Verification items for the finished model (mm, model axes). A direction names the side the tool comes from. Coordinates: 2 decimals unless noted, no trailing zeros. Order: outer loops, then holes, each group sorted by start corner. A loop starts at its lowest first (then second) coordinate and runs counter-clockwise, first axis right, second up. Notation, with made-up numbers: (-3, 35.5) -> (29, 35.5) arc R6 cw to (29, 45.5) -> close; hole circle Ø10 at (42, 59.5). An arc over 180 degrees is marked (long way). Write each question's results on one line, items separated by ' | '. Start each with the question number.
(1) Go/stop test with flat-tipped pins: pin 1 (2 mm diameter, centred on y = -5, z = -49, fed in from -X); pin 2 (2.5 mm diameter, centred on y = -3, z = -60.5, fed in from -X); pin 3 (2.5 mm diameter, centred on y = -5, z = -53, fed in from +X). Record where each tip stops, or that it passes through.
(2) Cross-section at D-D on z = -83.5. Enter the section's corners in (x, y), and give its area (3 significant figures).
(3) Cross-section at B-B on z = -15.5. Enter the section's corners in (x, y), and give its area (3 significant figures).
(4) Cross-section at C-C on x = -59.5. Enter the section's corners in (y, z).
(5) Cross-section at A-A on y = -4.25. Enter the section's corners in (x, z), and give its area (3 significant figures).
(6) Draft check along X on faces 3 (the flat face through (-15.492, -4, -57)), 4 (the cylindrical face through (-2.234, -3.757, -101.575)), 5 (the flat face through (1, -4, 0)). Enter one of: +X half, -X half, draft (parallel to the pull), parting line (faces both ways), or undercut.
(7) Thickness scan on probe 1 along X at (y, z) = (-2.25, -11.5); probe 2 along X at (y, z) = (-4.75, -36.5); probe 3 along Z at (x, y) = (20.5, -7). Record the ranges inside material, lowest first. Write a range as [from, to].
(8) Set-up check for faces 1 (the flat face through (29, -4, -43.686)), 2 (the flat face through (-1, -7.62, -39)): record each of +Z, -Z, +X, -X, +Y, -Y from which the full face is reachable in a straight line by a thin tool's end or side.
```python
from build123d import *

# Parameters (mm, degrees)
F1_DEPTH = 7.62


with BuildPart() as f1:
    # F0 (on Front) → F1 (new body)
    with BuildSketch(Plane.XZ):
        with BuildLine():
            Line((101.6, 0), (0, 0))
            Line((0, 0), (-101.6, 0))
            ThreePointArc((-101.6, 0), (0, -101.6), (101.6, 0))
        make_face()
        Polygon((22.649135, -66.423178), (0, -91.317579), (-22.649135, -66.423178), (-15.491997, -66.423178), (-15.491997, -47.441199), (0, -47.441199), (15.491997, -47.441199), (15.491997, -66.423178), align=None, mode=Mode.SUBTRACT)
        Polygon((-19.247199, -28.194), (-19.247199, -43.685997), (-38.229178, -43.685997), (-38.229178, -50.843135), (-63.123579, -28.194), (-38.229178, -5.544865), (-38.229178, -12.702003), (-19.247199, -12.702003), align=None, mode=Mode.SUBTRACT)
        Polygon((19.247199, -28.194), (19.247199, -12.702003), (38.229178, -12.702003), (38.229178, -5.544865), (63.123579, -28.194), (38.229178, -50.843135), (38.229178, -43.685997), (19.247199, -43.685997), align=None, mode=Mode.SUBTRACT)
    extrude(amount=F1_DEPTH)


solid = f1.part
```
Results are:
1) pin 1: stops at x = -89.55 | pin 2: stops at x = -82.53 | pin 3: stops at x = 87.43
2) outline: (-57.88, -7.62) -> (-7.11, -7.62) -> (-7.11, 0) -> (-57.88, 0) -> close; (7.11, -7.62) -> (57.88, -7.62) -> (57.88, 0) -> (7.11, 0) -> close | area: 774 mm2
3) outline: (-100.41, -7.62) -> (-49.17, -7.62) -> (-49.17, 0) -> (-100.41, 0) -> close; (-19.25, -7.62) -> (19.25, -7.62) -> (19.25, 0) -> (-19.25, 0) -> close; (49.17, -7.62) -> (100.41, -7.62) -> (100.41, 0) -> (49.17, 0) -> close | area: 1,070 mm2
4) outline: (-7.62, -82.35) -> (0, -82.35) -> (0, -31.49) -> (-7.62, -31.49) -> close; (-7.62, -24.9) -> (0, -24.9) -> (0, 0) -> (-7.62, 0) -> close
5) outline: (-101.6, 0) arc R101.6 ccw to (101.6, 0) -> close; hole (-63.12, -28.19) -> (-38.23, -50.84) -> (-38.23, -43.69) -> (-19.25, -43.69) -> (-19.25, -12.7) -> (-38.23, -12.7) -> (-38.23, -5.54) -> close; hole (-22.65, -66.42) -> (0, -91.32) -> (22.65, -66.42) -> (15.49, -66.42) -> (15.49, -47.44) -> (-15.49, -47.44) -> (-15.49, -66.42) -> close; hole (19.25, -43.69) -> (38.23, -43.69) -> (38.23, -50.84) -> (63.12, -28.19) -> (38.23, -5.54) -> (38.23, -12.7) -> (19.25, -12.7) -> close | area: 12,800 mm2
6) face 3: undercut | face 4: parting line | face 5: draft
7) probe 1: x = [-100.95, -44.77], [-38.23, 38.23], [44.77, 100.95] | probe 2: x = [-94.82, -53.99], [-19.25, 19.25], [53.99, 94.82] | probe 3: z = [-99.51, -68.79], [-66.42, -43.69], [-12.7, 0]
8) face 1: +Y, -Y | face 2: +Z, -Z, +X, -X, -Y
